Could you check a few things on this model? Use its own coordinates, in mm. A direction names the side the tool comes from. Coordinates: 2 decimals unless noted, no trailing zeros. Loops run counter-clockwise (first coordinate to the right, second up) from the corner with the lowest first, then second, coordinate; pieces in that order, holes last. Notation, with made-up numbers: (25, 38) -> (35, 38) arc R20 cw to (35, 71) -> close; hole circle Ø3 at (68, 76). An arc over 180 degrees is marked (long way). One line per question, with ' | ' between items.
```python
from build123d import *

# Parameters (mm, degrees)
F0_W        = 25.0751823187
F0_H        = 87.748773396
F1_DEPTH    = 57.4051365256
F2_T1_DEPTH = 214.0604270912
F3_R        = 5.08
F4_R        = 5.08
F5_W        = 10.9846293926
F5_H        = 22.9512043297
F6_DEPTH    = 76.7630785704
F7_R        = 5.08
F9_DEPTH    = 36.4525131881
F10_DEPTH   = 25.4


# Not quite as in the source:
# - a fillet or chamfer that OpenCascade refuses, or shapes differently, is made with other operations: its cross-section is extruded or revolved along the edge and cut away or added


with BuildPart() as f1:
    # F0 (on Top) → F1 (new body)
    with BuildSketch(Plane.XY):
        with Locations((12.5375911593, 10.7809714973)):
            Rectangle(F0_W, F0_H)
    extrude(amount=F1_DEPTH)

    # F2: fillet of radius 37.7970489545 on 2 edges, made by hand

    # F2_s2 → F2_t1 (cut)
    with BuildSketch(Plane.YZ.offset(-94.4926223863)):
        with BuildLine():
            ThreePointArc((-33.0934152007, 19.6080875711), (-22.0229158708, 46.3346371957), (4.7036337538, 57.4051365256))
            Line((4.7036337538, 57.4051365256), (-33.0934152007, 57.4051365256))
            Line((-33.0934152007, 57.4051365256), (-33.0934152007, 19.6080875711))
        make_face()
        with BuildLine():
            ThreePointArc((-33.0934152007, 37.7970489545), (-22.0229158708, 11.0704993299), (4.7036337538, 0))
            Line((4.7036337538, 0), (-33.0934152007, 0))
            Line((-33.0934152007, 0), (-33.0934152007, 37.7970489545))
        make_face()
    extrude(amount=F2_T1_DEPTH, mode=Mode.SUBTRACT)

    # F3
    f3_edges = [f1.edges().sort_by_distance(p)[0] for p in [
        (0, 29.679496, 0),
        (0, -18.586626, 8.028261),
        (25.075182, 29.679496, 57.405137),
        (25.075182, -18.586626, 49.376875),
        (25.075182, 29.679496, 0),
        (25.075182, -18.586626, 8.028261),
        (0, -18.586626, 49.376875),
        (0, 29.679496, 57.405137),
    ]]
    fillet(f3_edges, radius=F3_R)

    # F4
    f4_edges = [f1.edges().sort_by_distance(p)[0] for p in [
        (12.537591, -31.982976, 28.702568),
    ]]
    fillet(f4_edges, radius=F4_R)

    # F5 (on face) → F6 (cut)
    with BuildSketch(Plane(origin=(0, 0, 0), x_dir=(0, -1, 0), z_dir=(-1, 0, 0))):
        with Locations((-9.5620453358, 26.5463981777)):
            Rectangle(F5_W, F5_H)
    extrude(amount=-F6_DEPTH, mode=Mode.SUBTRACT)

    # F7
    f7_edges = [f1.edges().sort_by_distance(p)[0] for p in [
        (12.537591, 4.069731, 38.022),
        (12.537591, 4.069731, 15.070796),
        (12.537591, 15.05436, 15.070796),
        (12.537591, 15.05436, 38.022),
    ]]
    fillet(f7_edges, radius=F7_R)

    # F8 (on face) → F9 (join)
    with BuildSketch(Plane.XY.offset(57.4051365256)):
        Polygon((0, 18.3127000928), (5.08, 18.3127000928), (5.08, 41.8710074145), (0, 39.8706048727), align=None)
    extrude(amount=-F9_DEPTH)

    # F10 (add): a face of the model
    f10_faces = [f1.faces().sort_by_distance(p)[0] for p in [
        (11.2098476386, 29.6687845578, 57.4051365256),
    ]]
    extrude(f10_faces, amount=F10_DEPTH)


solid = f1.part
```
Q1. Imagine slicing it at C-C on y = 48.5. Write out the boundary of the cut face in (x, z).
Values follow:
outline: (0, 5.08) arc R5.08 ccw to (5.08, 0) -> (20, 0) arc R5.08 ccw to (25.08, 5.08) -> (25.08, 52.33) arc R5.08 ccw to (20, 57.41) -> (20, 82.81) -> (5.08, 82.81) -> (5.08, 57.41) arc R5.08 ccw to (0, 52.33) -> close
Q2. For pin 1 (4.5 mm diameter, centred on x = 12, z = 72, fed in from -Y); pin 2 (4 mm diameter, centred on y = 13.5, z = 67.5, fed in from -X); pin 3 (6 mm diameter, centred on x = 13.5, z = 57.5, fed in from -Y); pin 4 (5 mm diameter, centred on y = -12, z = 57.5, fed in from +X), each with a flat end and sliding along its axis, tell me the tip position at first contact or that it passes through.
Values follow:
pin 1: stops at y = 4.7 | pin 2: stops at x = 5.08 | pin 3: stops at y = -9.83 | pin 4: passes through
Q3. Please list where these lines run through material, in increasing order: L1, parallel to Y at x = 7, z = 71.5; L2, parallel to Z at x = 19.25, y = 11.5; L3, parallel to X at y = 10, z = 57.5. Write a range as [from, to].
Values follow:
L1: y = [4.7, 54.66] | L2: z = [0, 15.31], [37.79, 82.81] | L3: x = [5.08, 20]
Q4. Imagine slicing it at B-B on z = 66.5. Write out the boundary of the cut face in (x, y), plus the area to 3 significant figures.
Values follow:
outline: (0, 18.31) -> (5.08, 18.31) -> (5.08, 4.7) -> (20, 4.7) -> (20, 54.66) -> (5.08, 54.66) -> (5.08, 41.87) -> (0, 39.87) -> close | area: 860 mm2
Q5. Imagine slicing it at A-A on y = 12. Write out the boundary of the cut face in (x, z), plus the area to 3 significant figures.
Values follow:
outline: (0, 5.08) arc R5.08 ccw to (5.08, 0) -> (20, 0) arc R5.08 ccw to (25.08, 5.08) -> (25.08, 15.49) -> (0, 15.49) -> close; (0, 37.6) -> (25.08, 37.6) -> (25.08, 52.33) arc R5.08 ccw to (20, 57.41) -> (20, 82.81) -> (5.08, 82.81) -> (5.08, 57.41) arc R5.08 ccw to (0, 52.33) -> close | area: 1,240 mm2
Q6. We'd pull the mould along Z, two halves only. Please class faces 1 (the face through (0, 24, 35)), 2 (the face through (12, 15.054, 26)), 3 (the face through (1.449, 30.029, 1.528)), 4 (the face through (12.71, 13.53, 16.52)): released by +Z, released by -Z, zero draft, split by the parting line, or undercut.
Values follow:
face 1: zero draft | face 2: undercut | face 3: released by -Z | face 4: undercut
Q7. For faces 5 (the face through (12, 4.07, 26)), 6 (the face through (1.45, 47.37, 55.88)), 7 (the face through (3, 18.313, 71)), which set-ups out of +Z, -Z, +X, -X, +Y, -Y let a thin tool reach every point of the face, with its end or its side?
Values follow:
face 5: +X, -X | face 6: +Z, -X, +Y | face 7: +Z, -X, -Y
